Work out the finished part from the listing and answer in its coordinate system (mm). Face numbers are marked on the shaded views. A direction names the side the tool comes from. Coordinates: 2 decimals unless noted, no trailing zeros. Order: outer loops, then holes, each group sorted by start corner. A loop starts at its lowest first (then second) coordinate and runs counter-clockwise, first axis right, second up. Notation, with made-up numbers: M -29.75,7 L 3.25,7 A26 cw 3.25,21 Z; hole C 23,74.25 d7. An arc over 180 degrees is marked long. Use a Markdown table: item, result.
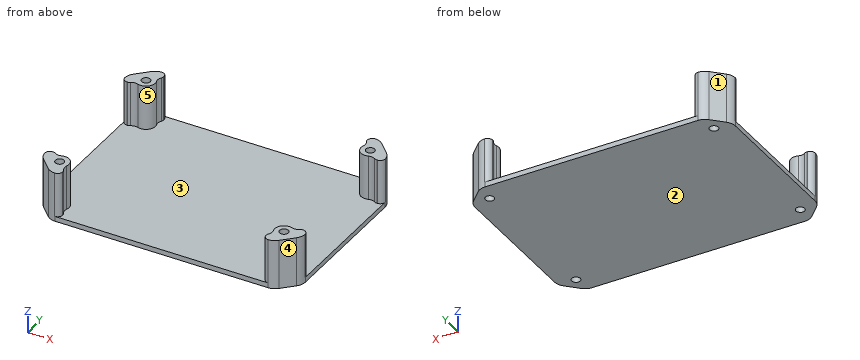
from build123d import *

# Parameters (mm, degrees)
EXTRUDE_1_DEPTH     = 20
SKETCH_2_R          = 1.75
CUT_EXTRUDE_1_DEPTH = 34
SHELL_1_T           = -2
FILLET_1_R          = 10
FILLET_2_R          = 3
FILLET_3_R          = 5
SKETCH_4_W          = 82
SKETCH_4_H          = 126.745531776
CUT_EXTRUDE_2_DEPTH = 18
FILLET_4_R          = 2
CUT_EXTRUDE_START   = -18
SKETCH_5_W          = 173.89587329
SKETCH_5_H          = 52
CUT_EXTRUDE_3_DEPTH = 18
FILLET_5_R          = 2


with BuildPart() as part:
    # Эскиз1 → Бобышка-Вытянуть1 (new body)
    with BuildSketch(Plane.XY):
        Polygon((-52.5, 30), (-45, 37.5), (45, 37.5), (52.5, 30), (52.5, -30), (45, -37.5), (-45, -37.5), (-52.5, -30), align=None)
    extrude(amount=EXTRUDE_1_DEPTH)

    # Эскиз2 → Вырез-Вытянуть1 (cut)
    with BuildSketch(Plane.XY.offset(20)):
        with Locations((-45.214466094, 30.214466094)):
            Circle(SKETCH_2_R)
        with Locations(Location((45.214466094, 30.214466094, 0), (0, 0, 180))):
            Circle(SKETCH_2_R)
        with Locations((45.214466094, -30.214466094)):
            Circle(SKETCH_2_R)
        with Locations(Location((-45.214466094, -30.214466094, 0), (0, 0, 180))):
            Circle(SKETCH_2_R)
    extrude(amount=-CUT_EXTRUDE_1_DEPTH, mode=Mode.SUBTRACT)

    # Оболочка1
    shell_1_openings = [part.faces().sort_by_distance(p)[0] for p in [
        (0, 0, 20),
    ]]
    offset(amount=SHELL_1_T, openings=shell_1_openings, kind=Kind.INTERSECTION)

    # Скругление1
    # the kernel refuses this fillet: 10 mm, written as the material it adds along each edge
    with BuildSketch(Plane(origin=(-45.74479618, -33.926776695, 2), x_dir=(0.7071067811865442, -0.7071067811865507, 0), z_dir=(0, 0, 1)), Plane(origin=(48.926776695, -30.74479618, 2), x_dir=(0.7071067811865482, 0.7071067811865467, 0), z_dir=(0, 0, 1)), Plane(origin=(45.74479618, 33.926776695, 2), x_dir=(-0.707106781186546, 0.7071067811865492, 0), z_dir=(0, 0, 1)), Plane(origin=(-48.926776695, 30.74479618, 2), x_dir=(-0.7071067811865508, -0.7071067811865444, 0), z_dir=(0, 0, 1))) as fillet_1_piece_1:
        with BuildLine():
            CenterArc((11.477032042, 3.794412555), FILLET_1_R, 183.312134334, 18.986942704)
            Line((1.493736012, 3.21665797), (1.294070091, 3.205102878))
            ThreePointArc((1.294070091, 3.205102878), (0.969771845, 1.504817982), (-0.12, 0.16))
            Line((-0.12, 0.16), (0, -0.2))
            ThreePointArc((0, -0.2), (1.112436867, -0.2), (2.039830568, -0.075888251))
            Line((2.039830568, -0.075888251), (2.224873734, 0))
        make_face()
    extrude(amount=18)
    with BuildSketch(Plane(origin=(-48.926776695, -30.74479618, 2), x_dir=(0.34351243985929386, 0.9391481265816991, 0), z_dir=(0, 0, 1)), Plane(origin=(45.74479618, -33.926776695, 2), x_dir=(-0.9391481265817004, 0.34351243985929, 0), z_dir=(0, 0, 1)), Plane(origin=(48.926776695, 30.74479618, 2), x_dir=(-0.3435124398592874, -0.9391481265817014, 0), z_dir=(0, 0, 1)), Plane(origin=(-45.74479618, 33.926776695, 2), x_dir=(0.9391481265817011, -0.34351243985928803, 0), z_dir=(0, 0, 1))) as fillet_1_piece_2:
        with BuildLine():
            CenterArc((8.275322434, 8.811292173), FILLET_1_R, 222.791938952, 18.986942704)
            Line((0.937067943, 2.017911495), (0.790302854, 1.882043882))
            ThreePointArc((0.790302854, 1.882043882), (0.287138375, 1.093191354), (-0.181395597, 0.084235607))
            Line((-0.181395597, 0.084235607), (0.094575114, -0.176225843))
            ThreePointArc((0.094575114, -0.176225843), (1.773283379, 0.245765435), (3.451991644, -0.176225843))
            Line((3.451991644, -0.176225843), (3.546566758, 0))
        make_face()
    extrude(amount=18)

    # Скругление2
    fillet_2_edges = [part.edges().sort_by_distance(p)[0] for p in [
        (-50.5, 29.171572875, 11),
        (-44.171572875, 35.5, 11),
        (-44.171572875, -35.5, 11),
        (-50.5, -29.171572875, 11),
        (44.171572875, -35.5, 11),
        (50.5, -29.171572875, 11),
        (50.5, 29.171572875, 11),
        (44.171572875, 35.5, 11),
    ]]
    fillet(fillet_2_edges, radius=FILLET_2_R)

    # Скругление3
    fillet_3_edges = [part.edges().sort_by_distance(p)[0] for p in [
        (45, 37.5, 10),
        (52.5, 30, 10),
        (52.5, -30, 10),
        (45, -37.5, 10),
        (-45, -37.5, 10),
        (-52.5, -30, 10),
        (-52.5, 30, 10),
        (-45, 37.5, 10),
    ]]
    fillet(fillet_3_edges, radius=FILLET_3_R)

    # Эскиз4 → Вырез-Вытянуть2 (cut)
    with BuildSketch(Plane.XY.offset(20)):
        Rectangle(SKETCH_4_W, SKETCH_4_H)
    extrude(amount=-CUT_EXTRUDE_2_DEPTH, mode=Mode.SUBTRACT)

    # Скругление4
    # the kernel refuses this fillet: 2 mm, written as the material it takes off along each edge
    with BuildSketch(Plane(origin=(41, -34.605706623, 2), x_dir=(0, -1, 0), z_dir=(0, 0, 1)), Plane(origin=(41, 34.605706623, 21.756559814), x_dir=(0, 1, 0), z_dir=(0, 0, -1))) as fillet_4_piece_1:
        with BuildLine():
            CenterArc((0.702623926, 2), FILLET_4_R, 235.828901177, 34.171098823)
            ThreePointArc((-0.420708294, 0.345272009), (-0.20250821, 0.18219615), (0, 0))
            Line((0, 0), (0.702623926, 0))
        make_face()
    extrude(amount=19.756559814, mode=Mode.SUBTRACT)
    with BuildSketch(Plane(origin=(41, -37.5, 25.118447555), x_dir=(0.9999997651545144, 0.0006853400003404547, 0), z_dir=(0, 0, -1)), Plane(origin=(-41, -37.5, 2), x_dir=(-0.9999997651545144, 0.0006853400003439418, 0), z_dir=(0, 0, 1)), Plane(origin=(41, 37.5, 2), x_dir=(0.9999997651545144, -0.0006853400003439394, 0), z_dir=(0, 0, 1))) as fillet_4_piece_2:
        with BuildLine():
            CenterArc((2.001370787, -1.999470741), FILLET_4_R, 88.681844886, 91.357422207)
            Line((0.001371257, -2.000841421), (-0.198628696, -2.000978489))
            Line((-0.198628696, -2.000978489), (-0.199999953, -0.000137068))
            Line((-0.199999953, -0.000137068), (-0.000137068, 0.199999953))
            ThreePointArc((-0.000137068, 0.199999953), (1.928794667, 0.201321927), (2.051979846, 0.199947074))
            Line((2.051979846, 0.199947074), (2.047379022, 0))
        make_face()
    extrude(amount=23.118447555, mode=Mode.SUBTRACT)
    with BuildSketch(Plane(origin=(-41, -34.605706623, 2), x_dir=(0, -1, 0), z_dir=(0, 0, 1))) as fillet_4_piece_3:
        with BuildLine():
            CenterArc((0.702623926, -2), FILLET_4_R, 90, 34.171098823)
            ThreePointArc((-0.420708294, -0.345272009), (-0.20250821, -0.18219615), (0, 0))
            Line((0, 0), (0.702623926, 0))
        make_face()
    extrude(amount=19.756559814, mode=Mode.SUBTRACT)
    with BuildSketch(Plane(origin=(-41, 34.605706623, 21.756559814), x_dir=(-0.6343994710236062, -0.7730053758965514, 0), z_dir=(0, 0, -1))) as fillet_4_piece_4:
        with BuildLine():
            CenterArc((0.72566687, 1.991754999), FILLET_4_R, 230.624541426, 34.171098823)
            Line((-0.543132072, 0.445744247), (0, 0))
            ThreePointArc((0, 0), (0.272125076, 0.012367502), (0.544250153, 0))
        make_face()
    extrude(amount=19.756559814, mode=Mode.SUBTRACT)
    with BuildSketch(Plane(origin=(-41, 37.5, 25.118447555), x_dir=(0, -1, 0), z_dir=(0, 0, -1))) as fillet_4_piece_5:
        with BuildLine():
            CenterArc((2.00084189, 2), FILLET_4_R, 178.642577793, 91.357422207)
            Line((0.001403151, 2.047378541), (-0.198540723, 2.052116395))
            ThreePointArc((-0.198540723, 2.052116395), (-0.2, 1.928932188), (-0.2, 0))
            Line((-0.2, 0), (0, -0.2))
            Line((0, -0.2), (2.00084189, -0.2))
            Line((2.00084189, -0.2), (2.00084189, 0))
        make_face()
    extrude(amount=23.118447555, mode=Mode.SUBTRACT)

    # Эскиз5 → Вырез-Вытянуть3 (cut)
    with BuildSketch(Plane.XY.offset(20).offset(CUT_EXTRUDE_START)):
        Rectangle(SKETCH_5_W, SKETCH_5_H)
    extrude(amount=CUT_EXTRUDE_3_DEPTH, mode=Mode.SUBTRACT)

    # Скругление5
    # the kernel refuses this fillet: 2 mm, written as the material it takes off along each edge
    with BuildSketch(Plane(origin=(49.605706623, -26, 21.756559814), x_dir=(1, 0, 0), z_dir=(0, 0, -1)), Plane(origin=(-49.605706623, -26, 2), x_dir=(-1, 0, 0), z_dir=(0, 0, 1))) as fillet_5_piece_1:
        with BuildLine():
            CenterArc((0.702623926, 2), FILLET_5_R, 235.828901177, 34.171098823)
            ThreePointArc((-0.420708294, 0.345272009), (-0.20250821, 0.18219615), (0, 0))
            Line((0, 0), (0.702623926, 0))
        make_face()
    extrude(amount=19.756559814, mode=Mode.SUBTRACT)
    with BuildSketch(Plane(origin=(52.5, -26, 25.118447555), x_dir=(-0.0006853400003439216, -0.9999997651545144, 0), z_dir=(0, 0, -1)), Plane(origin=(52.5, 26, 2), x_dir=(-0.0006853400003439287, 0.9999997651545144, 0), z_dir=(0, 0, 1)), Plane(origin=(-52.5, -26, 2), x_dir=(0.0006853400003439322, -0.9999997651545144, 0), z_dir=(0, 0, 1)), Plane(origin=(-52.5, 26, 25.118447555), x_dir=(0.0006853400003439264, 0.9999997651545144, 0), z_dir=(0, 0, -1))) as fillet_5_piece_2:
        with BuildLine():
            CenterArc((2.001370787, 1.999470741), FILLET_5_R, 179.960732907, 91.357422207)
            Line((0.001371257, 2.000841421), (-0.198628696, 2.000978489))
            Line((-0.198628696, 2.000978489), (-0.199999953, 0.000137068))
            Line((-0.199999953, 0.000137068), (-0.000137068, -0.199999953))
            ThreePointArc((-0.000137068, -0.199999953), (1.928794667, -0.201321927), (2.051979846, -0.199947074))
            Line((2.051979846, -0.199947074), (2.047379022, 0))
        make_face()
    extrude(amount=23.118447555, mode=Mode.SUBTRACT)
    with BuildSketch(Plane(origin=(49.605706623, 26, 21.756559814), x_dir=(-0.7730053758965525, 0.6343994710236047, 1.8308445150644594e-15), z_dir=(0, 0, -1))) as fillet_5_piece_3:
        with BuildLine():
            CenterArc((0.72566687, 1.991754999), FILLET_5_R, 230.624541426, 34.171098823)
            Line((-0.543132072, 0.445744247), (0, 0))
            ThreePointArc((0, 0), (0.272125076, 0.012367502), (0.544250153, 0))
        make_face()
    extrude(amount=19.756559814, mode=Mode.SUBTRACT)
    with BuildSketch(Plane(origin=(-49.605706623, 26, 2), x_dir=(-1, 0, 0), z_dir=(0, 0, 1))) as fillet_5_piece_4:
        with BuildLine():
            CenterArc((0.702623926, -2), FILLET_5_R, 90, 34.171098823)
            ThreePointArc((-0.420708294, -0.345272009), (-0.20250821, -0.18219615), (0, 0))
            Line((0, 0), (0.702623926, 0))
        make_face()
    extrude(amount=19.756559814, mode=Mode.SUBTRACT)


solid = part.part
(1) Straight lines are drawn through the part: L1, parallel to X at y = -29, z = 9.25; L2, parallel to Z at x = -2, y = 4; L3, parallel to X at y = -33, z = 11.25. For each, find the intervals that lie inside material, in ascending order.
Conclusion:
| item | result |
|---|---|
| L1 | -52.38 to -46.47, -43.95 to -41.67, 41.67 to 43.95, 46.47 to 52.38 |
| L2 | 0 to 2 |
| L3 | -49.5 to -41.82, 41.82 to 49.5 |
(2) A cutting plane is placed at B-B (z = 7.5). Give the number of separate pieces and of enclosed holes in the cut face, then the cut area to 3 significant figures.
Conclusion:
| item | result |
|---|---|
| separate pieces | 4 |
| enclosed holes | 4 |
| area | 318 mm2 |
(3) A cutting plane is placed at C-C (x = 0.5). Determine the outline of the cut face in (y, z).
Conclusion:
| item | result |
|---|---|
| outline | M -37.5,0 L 37.5,0 L 37.5,2 L -37.5,2 Z |
(4) Which of the six approach directions +Z, -Z, +X, -X, +Y, -Y give full straight-line access (tool end or side, diameter ignored) to the marked faces 4 and 5?
Conclusion:
| item | result |
|---|---|
| face 4 | +Z, -Z, +X, -Y |
| face 5 | +Z |
(5) A cutting plane is placed at A-A (y = 13.5). Determine the outline of the cut face in (x, z).
Conclusion:
| item | result |
|---|---|
| outline | M -52.5,0 L 52.5,0 L 52.5,2 L -52.5,2 Z |
(6) Determine the mould class of the marked faces 1, 2 and 3 for opening direction Y: pulls with the +Y half, pulls with the -Y half, needs draft (parallel to the pull), parting line crosses it, or undercut.
Conclusion:
| item | result |
|---|---|
| face 1 | pulls with the +Y half |
| face 2 | needs draft |
| face 3 | undercut |
(7) Given P1, Ø4, axis at y = 3, z = 4.5, coming from the -X side; P2, Ø1, axis at x = 41.5, z = 6.5, coming from the -Y side; P3, Ø1.5, axis at x = 7, y = 27, coming from the +Z side, each flat-ended and moving along its own axis, determine where each tip first touches the part or whether it passes through.
Conclusion:
| item | result |
|---|---|
| P1 | through |
| P2 | y = -37.23 |
| P3 | z = 2 |
